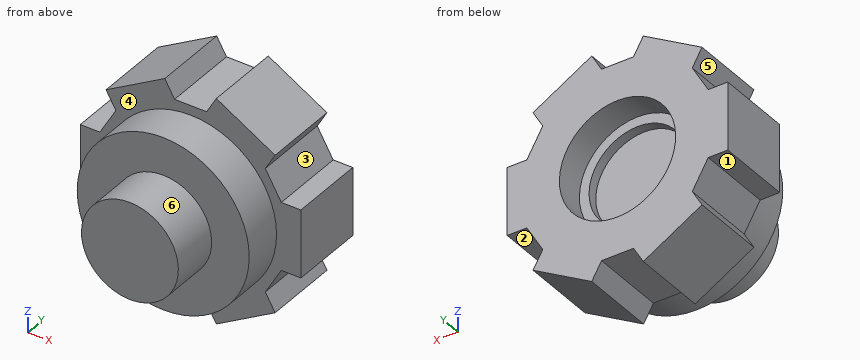
from build123d import *

# Parameters (mm, degrees)
SKETCH1_R           = 5
BOSS_EXTRUDE1_DEPTH = 5
SKETCH2_R           = 8.875
BOSS_EXTRUDE2_DEPTH = 4.11
BOSS_EXTRUDE3_DEPTH = 7.79
SKETCH4_R           = 6
CUT_EXTRUDE1_DEPTH  = 3
CUT_EXTRUDE2_START  = -1
SKETCH5_R           = 5
CUT_EXTRUDE2_DEPTH  = 1


with BuildPart() as part:
    # Sketch1 → Boss-Extrude1 (new body)
    with BuildSketch(Plane(origin=(0, 0, 0), x_dir=(1, 0, 0), z_dir=(0, 1, 0))):
        with Locations(Location((0, 0, 0), (0, 0, 270))):
            Circle(SKETCH1_R)
    extrude(amount=BOSS_EXTRUDE1_DEPTH)

    # Sketch2 → Boss-Extrude2 (add)
    with BuildSketch(Plane(origin=(0, 5, 0), x_dir=(1, 0, 0), z_dir=(0, 1, 0))):
        with Locations(Location((0, 0, 0), (0, 0, 270))):
            Circle(SKETCH2_R)
    extrude(amount=BOSS_EXTRUDE2_DEPTH)

    # Sketch3 → Boss-Extrude3 (add)
    with BuildSketch(Plane(origin=(0, 9.11, 0), x_dir=(1, 0, 0), z_dir=(0, 1, 0))):
        Polygon((9.364274058, 3.5), (11.385, 3.5), (11.385, -3.5), (9.364274058, -3.5), (7.713225942, -6.359699222), (8.723588913, -8.109699222), (2.661411087, -11.609699222), (1.651048116, -9.859699222), (-1.651048116, -9.859699222), (-2.661411087, -11.609699222), (-8.723588913, -8.109699222), (-7.713225942, -6.359699222), (-9.364274058, -3.5), (-11.385, -3.5), (-11.385, 3.5), (-9.364274058, 3.5), (-7.713225942, 6.359699222), (-8.723588913, 8.109699222), (-2.661411087, 11.609699222), (-1.651048116, 9.859699222), (1.651048116, 9.859699222), (2.661411087, 11.609699222), (8.723588913, 8.109699222), (7.713225942, 6.359699222), align=None)
    extrude(amount=BOSS_EXTRUDE3_DEPTH)

    # Sketch4 → Cut-Extrude1 (cut)
    with BuildSketch(Plane(origin=(0, 16.9, 0), x_dir=(1, 0, 0), z_dir=(0, 1, 0))):
        with Locations(Location((0, 0, 0), (0, 0, 270))):
            Circle(SKETCH4_R)
    extrude(amount=-CUT_EXTRUDE1_DEPTH, mode=Mode.SUBTRACT)

    # Sketch5 → Cut-Extrude2 (cut)
    with BuildSketch(Plane(origin=(0, 13.9, 0), x_dir=(1, 0, 0), z_dir=(0, 1, 0)).offset(CUT_EXTRUDE2_START)):
        with Locations(Location((0, 0, 0), (0, 0, 270))):
            Circle(SKETCH5_R)
    extrude(amount=CUT_EXTRUDE2_DEPTH, mode=Mode.SUBTRACT)


solid = part.part
Source: CAD feature listing. Evaluate the final solid. Frame: model axes, mm. Face numbers are marked on the shaded views. A direction names the side the tool comes from. Coordinates: 2 decimals unless noted, no trailing zeros. Loops run counter-clockwise (first coordinate to the right, second up) from the corner with the lowest first, then second, coordinate; pieces in that order, holes last. Notation, with made-up numbers: M 15,2 L 70,2 A29 cw 70,39 Z; hole C 87,17 d7. An arc over 180 degrees is marked long. Answer in a Markdown table with one row per item.
Q1. Ray query, probe 1 along X at (y, z) = (15.55, 0) (3 decimals); probe 2 along Y at (x, z) = (-2.5, -1.5); probe 3 along Y at (x, z) = (7.5, 8). Return the intervals inside material, ascending. Write a range as from..to.
Answers below:
| item | result |
|---|---|
| probe 1 | x = -11.385..-6, 6..11.385 |
| probe 2 | y = 0..12.9 |
| probe 3 | y = 9.11..16.9 |
Q2. Section A-A on z = 0. Return the cut outline in (x, y) (3 decimals), plus the area to 3 significant figures.
Answers below:
| item | result |
|---|---|
| outline | M -11.385,9.11 L -8.875,9.11 L -8.875,5 L -5,5 L -5,0 L 5,0 L 5,5 L 8.875,5 L 8.875,9.11 L 11.385,9.11 L 11.385,16.9 L 6,16.9 L 6,13.9 L 5,13.9 L 5,12.9 L -5,12.9 L -5,13.9 L -6,13.9 L -6,16.9 L -11.385,16.9 Z |
| area | 254 mm^2 |
Q3. Section C-C on x = 0. Return the cut outline in (y, z) (3 decimals).
Answers below:
| item | result |
|---|---|
| outline | M 0,-5 L 5,-5 L 5,-8.875 L 9.11,-8.875 L 9.11,-9.86 L 16.9,-9.86 L 16.9,-6 L 13.9,-6 L 13.9,-5 L 12.9,-5 L 12.9,5 L 13.9,5 L 13.9,6 L 16.9,6 L 16.9,9.86 L 9.11,9.86 L 9.11,8.875 L 5,8.875 L 5,5 L 0,5 Z |
Q4. Section B-B on y = 11.75. Return the cut outline in (x, z) (3 decimals).
Answers below:
| item | result |
|---|---|
| outline | M -11.385,-3.5 L -9.364,-3.5 L -7.713,-6.36 L -8.724,-8.11 L -2.661,-11.61 L -1.651,-9.86 L 1.651,-9.86 L 2.661,-11.61 L 8.724,-8.11 L 7.713,-6.36 L 9.364,-3.5 L 11.385,-3.5 L 11.385,3.5 L 9.364,3.5 L 7.713,6.36 L 8.724,8.11 L 2.661,11.61 L 1.651,9.86 L -1.651,9.86 L -2.661,11.61 L -8.724,8.11 L -7.713,6.36 L -9.364,3.5 L -11.385,3.5 Z |
Q5. Set-up query: the marked faces 1, 2 and 3. Return all of +Z, -Z, +X, -X, +Y, -Y with unobstructed straight access to the full face (end or side cutting, diameter ignored); none if empty.
Answers below:
| item | result |
|---|---|
| face 1 | -Z, -X, +Y, -Y |
| face 2 | -Z, +X, +Y, -Y |
| face 3 | +X, +Y, -Y |
Q6. Draft query along Z for the marked faces 4, 5 and 6. Return one class per face: pulls with the +Z half, pulls with the -Z half, needs draft (parallel to the pull), parting line crosses it, or undercut.
Answers below:
| item | result |
|---|---|
| face 4 | needs draft |
| face 5 | undercut |
| face 6 | parting line crosses it |
Q7. Section D-D on z = 7.75. Return the cut outline in (x, y).
Answers below:
| item | result |
|---|---|
| outline | M -8.52,9.11 L -4.32,9.11 L -4.32,5 L 4.32,5 L 4.32,9.11 L 8.52,9.11 L 8.52,16.9 L -8.52,16.9 Z |
Q8. First-contact query: pin 1 (13 mm diameter, centred on x = -2, z = -1.5, fed in from +Y); pin 2 (2.5 mm diameter, centred on x = 0.5, y = 12, fed in from -Z); pin 3 (1.6 mm diameter, centred on x = 10.5, y = 13.5, fed in from -Z); pin 4 (1 mm diameter, centred on y = 12, z = 4.5, fed in from +X). Flat tips, straight axial feed; report the tip coordinate or a pass-through.
Answers below:
| item | result |
|---|---|
| pin 1 | stops at y = 16.9 |
| pin 2 | stops at z = -10.03 |
| pin 3 | stops at z = -3.5 |
| pin 4 | stops at x = 9.08 |
